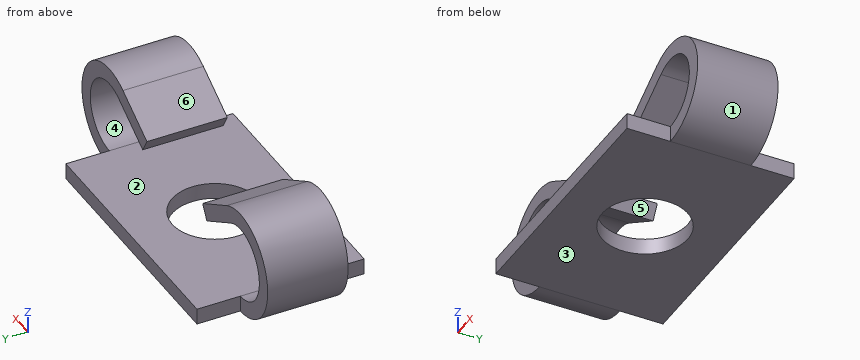
from build123d import *

# Parameters (mm, degrees)
SKETCH_1_W      = 23.5
SKETCH_1_H      = 15.6
SKETCH_1_R      = 4
EXTRUDE_1_DEPTH = 1.5
EXTRUDE_2_DEPTH = 3.75


with BuildPart() as part:
    # Эскиз1 → Бобышка-Вытянуть1 (new body)
    with BuildSketch(Plane.XY):
        Rectangle(SKETCH_1_W, SKETCH_1_H)
        Circle(SKETCH_1_R, mode=Mode.SUBTRACT)
    extrude(amount=EXTRUDE_1_DEPTH)

    # Эскиз3 → Бобышка-Вытянуть2 (add, symmetric)
    with BuildSketch(Plane(origin=(0, 0, 0), x_dir=(1, 0, 0), z_dir=(0, 1, 0))):
        with BuildLine():
            Line((-10.05, -7.844486373), (-5.75, -5.361880215))
            Line((-5.75, -5.361880215), (-5, -6.660918321))
            Line((-5, -6.660918321), (-9.3, -9.143524479))
            ThreePointArc((-9.3, -9.143524479), (-16.483036549, -6.168213321), (-11.75, 0))
            Line((-11.75, 0), (-11.75, -1.5))
            ThreePointArc((-11.75, -1.5), (-15.034147809, -5.779984753), (-10.05, -7.844486373))
        make_face()
    extrude_2 = extrude(amount=EXTRUDE_2_DEPTH, both=True)

    # Зеркальное отражение1: Бобышка-Вытянуть2 across plane
    add(extrude_2.mirror(Plane(origin=(0, 0, 0), x_dir=(0, 0, 1), z_dir=(1, 0, 0))))


solid = part.part
Verification items for the finished model (mm, model axes). Face numbers are marked on the shaded views. A direction names the side the tool comes from. Coordinates: 2 decimals unless noted, no trailing zeros. Loops run counter-clockwise (first coordinate to the right, second up) from the corner with the lowest first, then second, coordinate; pieces in that order, holes last. Notation, with made-up numbers: M -16,22 L 30,22 A20 ccw 30,29 Z; hole C 57,70.25 d5. An arc over 180 degrees is marked long. One line per item, written item: value.
1. Section check B-B on x = 8. Record the cut outline in (y, z), plus the area to 3 significant figures.
Answers follow:
outline: M -7.8,0 L 7.8,0 L 7.8,1.5 L -7.8,1.5 Z; M -3.75,6.66 L 3.75,6.66 L 3.75,8.39 L -3.75,8.39 Z
area: 36.4 mm^2
2. Material ranges on line 1 along X through (y, z) = (-0.5, 4.9); line 2 along Z through (x, y) = (-11.75, -1.5); line 3 along X through (y, z) = (-0.25, 7.75), recorded low to high. Write a range as from..to.
Answers follow:
line 1: -16.65..-15.15, 15.15..16.65
line 2: 0..1.5, 8.3..9.8
line 3: -15.74..-13.6, -9.89..-6.89, 6.89..9.89, 13.6..15.74
3. Mould release check, pull along Z, two halves, no side actions. Record for the marked faces 1, 2, 3 and 4: pulls with the +Z half, pulls with the -Z half, needs draft (parallel to the pull), parting line crosses it, or undercut.
Answers follow:
face 1: parting line crosses it
face 2: undercut
face 3: pulls with the -Z half
face 4: undercut
4. Section check A-A on z = 4.9. Record the cut outline in (x, y).
Answers follow:
outline: M -16.65,-3.75 L -15.15,-3.75 L -15.15,3.75 L -16.65,3.75 Z; M 15.15,-3.75 L 16.65,-3.75 L 16.65,3.75 L 15.15,3.75 Z
5. Section check D-D on z = 6.25. Record the cut outline in (x, y), plus the area to 3 significant figures.
Answers follow:
outline: M -16.46,-3.75 L -14.87,-3.75 L -14.87,3.75 L -16.46,3.75 Z; M -7.29,-3.75 L -5.24,-3.75 L -5.24,3.75 L -7.29,3.75 Z; M 5.24,-3.75 L 7.29,-3.75 L 7.29,3.75 L 5.24,3.75 Z; M 14.87,-3.75 L 16.46,-3.75 L 16.46,3.75 L 14.87,3.75 Z
area: 54.6 mm^2
6. Section check C-C on y = 0. Record the cut outline in (x, z), plus the area to 3 significant figures.
Answers follow:
outline: M -11.75,0 L -4,0 L -4,1.5 L -11.75,1.5 A3.4 cw long -10.05,7.84 L -5.75,5.36 L -5,6.66 L -9.3,9.14 A4.9 ccw long Z; M 4,0 L 11.75,0 A4.9 ccw long 9.3,9.14 L 5,6.66 L 5.75,5.36 L 10.05,7.84 A3.4 cw long 11.75,1.5 L 4,1.5 Z
area: 83.8 mm^2
7. Gauge pin test, flat ends, axial feed: P1, Ø0.8, axis at y = 5.5, z = 1, coming from the -X side; P2, Ø4, axis at x = 9.5, y = -6, coming from the +Z side; P3, Ø4, axis at y = -3, z = 8, coming from the -X side. Record the tip position at first contact, or that the pin passes through.
Answers follow:
P1: x = -11.75
P2: z = 1.5
P3: x = -16.52
8. Set-up check for the marked faces 5 and 6: record each of +Z, -Z, +X, -X, +Y, -Y from which the full face is reachable in a straight line by a thin tool's end or side.
Answers follow:
face 5: +Y, -Y
face 6: +Z, +Y, -Y
